Check sheet for the modelled part. Datum: model origin and axes. Units: mm. A direction names the side the tool comes from. Coordinates: 2 decimals unless noted, no trailing zeros. Order: outer loops, then holes, each group sorted by start corner. A loop starts at its lowest first (then second) coordinate and runs counter-clockwise, first axis right, second up.
Autodesk Inventor part; units mm, degrees
ref_plane "YZ Plane" through (0, 0, 0) normal (1, 0, 0) x (0, 1, 0)
ref_plane "XZ Plane" through (0, 0, 0) normal (0, 1, 0) x (-1, 0, 0)
ref_plane "XY Plane" through (0, 0, 0) normal (0, 0, 1) x (1, 0, 0)
sketch "Sketch1" plane through (0, 0, 0) normal (0, 1, 0) x (-1, 0, 0)
  line L0 (-166.6875, -59.5312) -> (166.6875, -59.5312)
  line L1 (166.6875, -59.5312) -> (166.6875, 59.5312)
  line L2 (166.6875, 59.5312) -> (-166.6875, 59.5312)
  line L3 (-166.6875, 59.5312) -> (-166.6875, -59.5312)
  line L4 (-166.6875, -59.5312) -> (166.6875, 59.5312) construction
  line L5 (166.6875, -59.5312) -> (-166.6875, 59.5312) construction
  point P0 (0, 0)
  point P1 (0, 0)
  dimension "d0" = 333.375
  dimension "d1" = 119.0625
extrude "Extrusion1" add sketch "Sketch1" along normal blind 88.9
sketch "Sketch2" plane through (0, 88.9, 0) normal (0, 1, 0) x (1, 0, 0)
  line L0 (166.6875, 59.5312) -> (-166.6875, 59.5312)
  line L1 (-166.6875, 59.5312) -> (-166.6875, -59.5312)
  line L2 (-166.6875, -59.5312) -> (166.6875, -59.5312)
  line L3 (166.6875, -59.5312) -> (166.6875, 59.5312)
  line L4 (-147.6375, 40.4812) -> (147.6375, 40.4812)
  line L5 (147.6375, 40.4812) -> (147.6375, -40.4812)
  line L6 (147.6375, -40.4812) -> (-147.6375, -40.4813)
  line L7 (-147.6375, -40.4813) -> (-147.6375, 40.4812)
  point P0 (0, 0)
  dimension "d4" = 19.05
  dimension "d5" = 19.05
  dimension "d6" = 19.05
  dimension "d7" = 19.05
extrude "Extrusion2" cut sketch "Sketch2" against normal through all contours L4 L5 L6 L7
sketch "Sketch3" plane through (166.6875, 0, -59.5312) normal (0, 0, -1) x (-1, 0, 0)
  line L0 (0, 88.9) -> (333.375, 0) construction
  line L1 (0, 0) -> (333.375, 88.9) construction
  point P0 (166.6875, 0)
  point P1 (166.6875, 44.45)
hole "Hole1" at (0, 44.45, -59.5312) direction (0, 0, 1) diameter 11.9062 end through all
sketch "Sketch4" plane through (166.6875, 0, 59.5312) normal (1, 0, 0) x (0, 0, -1)
  line L0 (0, 0) -> (119.0625, 88.9) construction
  line L1 (0, 88.9) -> (119.0625, 0) construction
  point P0 (59.5312, 0)
  point P1 (59.5312, 44.45)
hole "Hole2" at (166.6875, 44.45, 0) direction (-1, 0, 0) diameter 11.9062 end through all
sketch "Sketch5" plane through (0, 88.9, 0) normal (0, 1, 0) x (1, 0, 0)
  line L0 (-147.6375, -40.4813) -> (-147.6375, 40.4812)
  line L1 (-147.6375, 40.4812) -> (147.6375, 40.4812)
  line L2 (147.6375, 40.4812) -> (147.6375, -40.4812)
  line L3 (147.6375, -40.4812) -> (-147.6375, -40.4813)
  line L4 (166.6875, 59.5312) -> (-166.6875, 59.5312)
  line L5 (-166.6875, 59.5312) -> (-166.6875, -59.5312)
  line L6 (-166.6875, -59.5312) -> (166.6875, -59.5312)
  line L7 (166.6875, -59.5312) -> (166.6875, 59.5312)
  line L8 (0, 59.5312) -> (0, -59.5312) construction
  point P0 (0, 0)
equation "\"d5\" = d4"
equation "\"d6\" = d4"
equation "\"d7\" = d4"
properties part number "gyroWheelCradle01" material "Wood (Maple)"
(1) Cross-section at C-C (z = 0). Enter the section's corners in (x, y).
Filled in:
outline: (-166.69, 0) - (-147.64, 0) - (-147.64, 38.5) - (-166.69, 38.5) - close; (-166.69, 50.4) - (-147.64, 50.4) - (-147.64, 88.9) - (-166.69, 88.9) - close; (147.64, 0) - (166.69, 0) - (166.69, 38.5) - (147.64, 38.5) - close; (147.64, 50.4) - (166.69, 50.4) - (166.69, 88.9) - (147.64, 88.9) - close
(2) Thickness scan on probe 1 along X at (y, z) = (70, 28); probe 2 along Z at (x, y) = (22, 56.5); probe 3 along X at (y, z) = (44.45, 46). Record the ranges inside material, lowest first.
Filled in:
probe 1: x = -166.69 to -147.64, 147.64 to 166.69
probe 2: z = -59.53 to -40.48, 40.48 to 59.53
probe 3: x = -166.69 to -5.95, 5.95 to 166.69
(3) Release check for a two-part mould opening along Y. For faces 1 (the cylindrical face through (-1.788, 50.128, -49.873)), 2 (the flat face through (39, 0, 41)), 3 (the flat face through (39, 88.9, 41)) record: +Y half, -Y half, draft (parallel to the pull), parting line (faces both ways), or undercut.
Filled in:
face 1: undercut
face 2: -Y half
face 3: +Y half
(4) Cross-section at B-B (y = 44.45). Enter the section's corners in (x, z), and give its area (3 significant figures).
Filled in:
outline: (-166.69, -59.53) - (-5.95, -59.53) - (-5.95, -40.48) - (-147.64, -40.48) - (-147.64, -5.95) - (-166.69, -5.95) - close; (-166.69, 5.95) - (-147.64, 5.95) - (-147.64, 40.48) - (-5.95, 40.48) - (-5.95, 59.53) - (-166.69, 59.53) - close; (5.95, -59.53) - (166.69, -59.53) - (166.69, -5.95) - (147.64, -5.95) - (147.64, -40.48) - (5.95, -40.48) - close; (5.95, 40.48) - (147.64, 40.48) - (147.64, 5.95) - (166.69, 5.95) - (166.69, 59.53) - (5.95, 59.53) - close
area: 14,900 mm2
(5) Cross-section at D-D (x = 0). Enter the section's corners in (y, z).
Filled in:
outline: (0, -59.53) - (38.5, -59.53) - (38.5, -40.48) - (0, -40.48) - close; (0, 40.48) - (38.5, 40.48) - (38.5, 59.53) - (0, 59.53) - close; (50.4, -59.53) - (88.9, -59.53) - (88.9, -40.48) - (50.4, -40.48) - close; (50.4, 40.48) - (88.9, 40.48) - (88.9, 59.53) - (50.4, 59.53) - close
(6) Go/stop test with a flat-tipped pin: P1, Ø9.5, axis at y = 44.45, z = 0, coming from the -X side. Record where the tip stops, or that it passes through.
Filled in:
P1: passes through
(7) Cross-section at A-A (x = 144.5). Enter the section's corners in (y, z), and give its area (3 significant figures).
Filled in:
outline: (0, -59.53) - (88.9, -59.53) - (88.9, -40.48) - (0, -40.48) - close; (0, 40.48) - (88.9, 40.48) - (88.9, 59.53) - (0, 59.53) - close
area: 3,390 mm2
(8) Tool access check on faces 4 (the flat face through (147.638, 45, 8)), 5 (the flat face through (-166.688, 34, -1)). Record the directions out of +Z, -Z, +X, -X, +Y, -Y that give a thin tool (end or side, any length) a straight path to the whole face; none if there is none.
Filled in:
face 4: +Y, -Y
face 5: +Z, -Z, -X, +Y, -Y
